from build123d import *

# Parameters (mm, degrees)
SKETCH1_R           = 75
SKETCH1_R_2         = 70
BOSS_EXTRUDE1_DEPTH = 100


with BuildPart() as part:
    # Sketch1 → Boss-Extrude1 (new body)
    with BuildSketch(Plane(origin=(0, 0, 0), x_dir=(1, 0, 0), z_dir=(0, 1, 0))):
        with Locations(Location((0, 0, 0), (0, 0, 270))):
            Circle(SKETCH1_R)
        with Locations(Location((0, 0, 0), (0, 0, 270))):
            Circle(SKETCH1_R_2, mode=Mode.SUBTRACT)
    extrude(amount=BOSS_EXTRUDE1_DEPTH)

    # Sketch3 → Revolve1 (revolve)
    with BuildSketch(Plane(origin=(0, 0, 0), x_dir=(0, 0, -1), z_dir=(1, 0, 0)), mode=Mode.PRIVATE) as revolve1_sk:
        with BuildLine():
            Line((-70, 100), (-75, 100))
            Line((-75, 100), (-75, 105))
            add(Edge.make_bspline(
                [(-20, 130), (-50.667187392, 123.477390111), (-75, 105)],
                knots=[0, 0, 0, 1, 1, 1], degree=2))
            Line((-20, 130), (0, 130))
            Line((0, 130), (0, 122.928932188))
            Line((0, 122.928932188), (-20, 122.928932188))
            add(Edge.make_bspline(
                [(-20, 122.928932188), (-48.64448062, 117.780957156), (-70, 100)],
                knots=[0, 0, 0, 1, 1, 1], degree=2))
        make_face()
    revolve(revolve1_sk.sketch.rotate(Axis((0, -20.154872571, 0), (0, 1, 0)), 180), axis=Axis((0, -20.154872571, 0), (0, 1, 0)))


solid = part.part
Could you check a few things on this model? Use its own coordinates, in mm. A direction names the side the tool comes from. Give positions to 0.01 mm unless a question says otherwise; leave off trailing zeros. Order: outer loops, then holes, each group sorted by start corner. A loop starts at its lowest first (then second) coordinate and runs counter-clockwise, first axis right, second up.
1. Suppose I cut it at A-A (y = 44). Write out the boundary of the cut face in (x, z).
Answers below:
outline: circle Ø150 at (0, 0); hole circle Ø140 at (0, 0)
2. I need wall thicknesses on L1, parallel to X at y = 30.5, z = 0; L2, parallel to Z at x = -41, y = 56; L3, parallel to X at y = 14.5, z = 15.5. Which ranges of each line are inside material? Lowest first, please.
Answers below:
L1: x = -75 to -70, 70 to 75
L2: z = -62.8 to -56.74, 56.74 to 62.8
L3: x = -73.38 to -68.26, 68.26 to 73.38
3. Which directions (+Z, -Z, +X, -X, +Y, -Y) give clear straight access to the entire face, cutting with the end or side of a thin tool? Please do faces 1 (the flat face through (0, 122.929, 0)), 2 (the flat face through (0, 130, 0)).
Answers below:
face 1: -Y
face 2: +Z, -Z, +X, -X, +Y
4. For pin 1 (2 mm diameter, centred on x = -52.5, y = 28, fed in from -Z); pin 2 (3 mm diameter, centred on x = 39, z = -41, fed in from +Y); pin 3 (20 mm diameter, centred on x = 10, z = -2, fed in from -Y), each with a flat end and sliding along its axis, tell me the tip position at first contact or that it passes through.
Answers below:
pin 1: stops at z = -54.52
pin 2: stops at y = 117.58
pin 3: stops at y = 122.89
5. Thinking about a two-plate mould opening in Z: for faces 3 (the flat face through (-50, 0, 50)), 4 (the cylindrical face through (-42.594, 49.3, -55.55)), which applies, +Z half, -Z half, draft (parallel to the pull), parting line (faces both ways), or undercut?
Answers below:
face 3: draft
face 4: undercut
